Autodesk Inventor part; units mm, degrees
ref_plane "YZ Plane" through (0, 0, 0) normal (1, 0, 0) x (0, 1, 0)
ref_plane "XZ Plane" through (0, 0, 0) normal (0, 1, 0) x (-1, 0, 0)
ref_plane "XY Plane" through (0, 0, 0) normal (0, 0, 1) x (1, 0, 0)
sketch "草图1" plane through (0, 0, 0) normal (0, 1, 0) x (-1, 0, 0)
  circle A0 centre (0, 0) radius 15
  circle A1 centre (0, 0) radius 10
  line L0 (0, 20.4744) -> (0, -21.3556)
  dimension "d0" = 30
  dimension "d1" = 20
extrude "拉伸1" add sketch "草图1" along normal blind 20 contours A0 L0 A1 | L0 A1 A0
sketch "草图2" plane through (0, 20, 0) normal (0, 1, 0) x (1, 0, 0)
  circle A0 centre (0, 0) radius 15
  line L0 (-5, 17.5) -> (5, 17.5)
  line L1 (5, 17.5) -> (5, -17.5)
  line L2 (5, -17.5) -> (-5, -17.5)
  line L3 (-5, -17.5) -> (-5, 17.5)
  line L4 (-5, 17.5) -> (5, -17.5) construction
  line L5 (5, 17.5) -> (-5, -17.5) construction
  dimension "d5" = 10
  dimension "d6" = 35
extrude "拉伸2" cut sketch "草图2" against normal blind 5 contours L1 A0 L3 | A0 L3 L0 L1 | L1 L2 L3 A0
sketch "草图3" plane through (0, 0, 0) normal (0, -1, 0) x (1, 0, 0)
  circle A0 centre (0, 0) radius 10
  circle A1 centre (0, 0) radius 15
  arc A2 (-22.5, 8) -> (-22.5, -8) centre (-22.5, 0) ccw
  line L0 (-22.5, 8) -> (-12.6886, 8)
  line L1 (-22.5, -8) -> (-12.6886, -8)
  circle A3 centre (22.5, 0) radius 4
  circle A4 centre (-22.5, 0) radius 4
  line L2 (0, 19.1751) -> (0, -20.0629)
  arc A5 (22.5, -8) -> (22.5, 8) centre (22.5, 0) ccw
  line L3 (22.5, 8) -> (12.6886, 8)
  line L4 (22.5, -8) -> (12.6886, -8)
  dimension "d10" = 16
  dimension "d11" = 8
  dimension "d12" = 16
  dimension "d13" = 45
  dimension "d14" = 22.5
extrude "拉伸3" add sketch "草图3" against normal blind 6 contours L3 A5 L4 A1 | A1 L1 A2 L0
For this review, take the finished solid that the model builds, in its own axes (mm). A direction names the side the tool comes from. Coordinates: 2 decimals unless noted, no trailing zeros. Write each loop counter-clockwise with the first axis right and the second up, starting at its lowest first coordinate (ties: lowest second). Pieces come first, ordered by that corner, then holes.
(1) Add section C-C on y = 17.5. Give the boundary of the cut face in (x, z), then the cut area to 3 significant figures.
(2) Add section D-D on z = 6.25. Give the boundary of the cut face in (x, y), then the cut area to 3 significant figures.
(3) Add section A-A on x = 0. Give the boundary of the cut face in (y, z).
(4) Add section B-B on z = 0. Give the boundary of the cut face in (x, y).
(5) Tool access review of faces 1 (the face through (18, 3, 8)), 2 (the face through (-18, 3, -8)), 3 (the face through (14.985, 9.86, -0.66)), 4 (the face through (-18, 3, 8)), 5 (the face through (0, 15, -12)): name each direction out of +Z, -Z, +X, -X, +Y, -Y from which nothing blocks a thin tool from reaching the whole face with its end or side.
(6) Wall thickness on probe 1 along Z at (x, y) = (22.5, 3.7); probe 2 along Y at (x, z) = (-26, -7); probe 3 along X at (y, z) = (17.75, 3.5): over which ranges is each line inside the solid? List them lowest first.
(7) For pin 1 Ø4 at (y, z) = (12, 11.5) entering from -X; pin 2 Ø8 at (x, y) = (6, 8) entering from +Z; pin 3 Ø1 at (y, z) = (5.5, -7) entering from +X, all flat-tipped, find the tip position at first contact; note any pin that passes through.
(8) The part is to be moulded in two halves that separate along X. For faces 6 (the face through (-25.7, 3, -2.4)), 7 (the face through (18, 3, -8)), 8 (the face through (30.498, 2.958, -0.176)), say which applies: +X half, -X half, draft (parallel to the pull), parting line (faces both ways), or undercut.
Answer sheet:
1. outline: (-5, -14.14) - (-5, -8.66) arc R10 cw to (-5, 8.66) - (-5, 14.14) arc R15 ccw to start; (5, -14.14) arc R15 ccw to (5, 14.14) - (5, 8.66) arc R10 cw to (5, -8.66) - close
1. area: 290 mm2
2. outline: (-27.49, 0) - (-7.81, 0) - (-7.81, 20) - (-13.64, 20) - (-13.64, 6) - (-27.49, 6) - close; (7.81, 0) - (27.49, 0) - (27.49, 6) - (13.64, 6) - (13.64, 20) - (7.81, 20) - close
2. area: 399 mm2
3. outline: (0, -15) - (15, -15) - (15, -10) - (0, -10) - close; (0, 10) - (15, 10) - (15, 15) - (0, 15) - close
4. outline: (-30.5, 0) - (-26.5, 0) - (-26.5, 6) - (-30.5, 6) - close; (-18.5, 0) - (-10, 0) - (-10, 20) - (-15, 20) - (-15, 6) - (-18.5, 6) - close; (10, 0) - (18.5, 0) - (18.5, 6) - (15, 6) - (15, 20) - (10, 20) - close; (26.5, 0) - (30.5, 0) - (30.5, 6) - (26.5, 6) - close
5. face 1: +Z, +X, +Y, -Y
5. face 2: -Z, -X, +Y, -Y
5. face 3: +Y
5. face 4: +Z, -X, +Y, -Y
5. face 5: +Z, -Z, +Y
6. probe 1: z = -8 to -4, 4 to 8
6. probe 2: y = 0 to 6
6. probe 3: x = -14.59 to -9.37, 9.37 to 14.59
7. pin 1: stops at x = -11.61
7. pin 2: stops at z = 14.87
7. pin 3: stops at x = 27.16
8. face 6: undercut
8. face 7: draft
8. face 8: +X half
